```python
from build123d import *

# Parameters (mm, degrees)
PAD_DEPTH         = 27
SKETCH001_R       = 1.6
POCKET_DEPTH      = 14.501
POCKET_DEPTH_BACK = -14.501


with BuildPart() as part:
    # Sketch → Pad (new body, symmetric)
    with BuildSketch(Plane.XZ):
        Polygon((-14.5, 14.1), (-14.5, 0), (14.5, 0), (14.5, 14.1), (12.95, 14.1), (12.95, 1.2), (-12.95, 1.2), (-12.95, 14.1), align=None)
    extrude(amount=PAD_DEPTH, both=True)

    # Sketch001 → Pocket (cut, two sides)
    with BuildSketch(Plane.YZ) as pocket_sk:
        with Locations((-12.5, 9.1)):
            Circle(SKETCH001_R)
        with Locations((12.5, 9.1)):
            Circle(SKETCH001_R)
    extrude(amount=-POCKET_DEPTH, mode=Mode.SUBTRACT)
    extrude(pocket_sk.sketch, amount=-POCKET_DEPTH_BACK, mode=Mode.SUBTRACT)


solid = part.part
```
The listing builds one solid part. Answer for the finished solid, in the listing's coordinates (mm). A direction names the side the tool comes from. Round coordinates to 2 decimals unless told otherwise and drop trailing zeros. Order: outer loops, then holes, each group sorted by start corner. A loop starts at its lowest first (then second) coordinate and runs counter-clockwise, first axis right, second up. Notation, with made-up numbers: (59, -4) -> (74, -4) arc R30 cw to (74, 32) -> close; hole circle Ø5 at (35, 87.5). An arc over 180 degrees is marked (long way). Answer as CSV lines item,"result". Start each with the question number.
(1) A tool of negligible diameter and unlimited length cuts with its end or side. For faces 4 (the face through (0, 0, 1.2)), 5 (the face through (-2, -27, 1)), from which of +Z, -Z, +X, -X, +Y, -Y can it reach the whole face along a straight path? Write none if from no direction.
(2) For a pull along X with two mould halves and no side action, classify faces 1 (the face through (-14, 0, 14.1)), 2 (the face through (12.95, 0, 8)), 3 (the face through (-14.5, 0, 7)) as +X half, -X half, draft (parallel to the pull), parting line (faces both ways), or undercut.
(3) The part is cut by section D-D (x = 11.25). Determine the outline of the cut face in (y, z), then the cut area to 3 significant figures.
(4) The part is cut by section A-A (z = 9.1). Determine the outline of the cut face in (x, y), then the cut area to 3 significant figures.
(5) Find the intervals of material crossed by probe 1 along Y at (x, z) = (13.7, 9.1); probe 2 along X at (y, z) = (19, 5); probe 3 along Z at (x, y) = (13.5, -12.5), in increasing order. Write a range as from..to.
(6) A flat-ended cylindrical pin translates along its axis: pin 1 Ø1.5 at (x, y) = (-5.5, -13) entering from +Z. Find the tip coordinate at first contact, or state that the pin passes through.
(7) The part is cut by section C-C (y = 4). Determine the outline of the cut face in (x, z), then the cut area to 3 significant figures.
(8) The part is cut by section B-B (y = 12.5). Determine the outline of the cut face in (x, z).
Evaluation:
1,face 4,"+Z, +Y, -Y"
1,face 5,"+Z, -Z, +X, -X, -Y"
2,face 1,"draft"
2,face 2,"undercut"
2,face 3,"-X half"
3,outline,"(-27, 0) -> (27, 0) -> (27, 1.2) -> (-27, 1.2) -> close"
3,area,"64.8 mm²"
4,outline,"(-14.5, -27) -> (-12.95, -27) -> (-12.95, -14.1) -> (-14.5, -14.1) -> close; (-14.5, -10.9) -> (-12.95, -10.9) -> (-12.95, 10.9) -> (-14.5, 10.9) -> close; (-14.5, 14.1) -> (-12.95, 14.1) -> (-12.95, 27) -> (-14.5, 27) -> close; (12.95, -27) -> (14.5, -27) -> (14.5, -14.1) -> (12.95, -14.1) -> close; (12.95, -10.9) -> (14.5, -10.9) -> (14.5, 10.9) -> (12.95, 10.9) -> close; (12.95, 14.1) -> (14.5, 14.1) -> (14.5, 27) -> (12.95, 27) -> close"
4,area,"148 mm²"
5,probe 1,"-27..-14.1, -10.9..10.9, 14.1..27"
5,probe 2,"-14.5..-12.95, 12.95..14.5"
5,probe 3,"0..7.5, 10.7..14.1"
6,pin 1,"z = 1.2"
7,outline,"(-14.5, 0) -> (14.5, 0) -> (14.5, 14.1) -> (12.95, 14.1) -> (12.95, 1.2) -> (-12.95, 1.2) -> (-12.95, 14.1) -> (-14.5, 14.1) -> close"
7,area,"74.8 mm²"
8,outline,"(-14.5, 0) -> (14.5, 0) -> (14.5, 7.5) -> (12.95, 7.5) -> (12.95, 1.2) -> (-12.95, 1.2) -> (-12.95, 7.5) -> (-14.5, 7.5) -> close; (-14.5, 10.7) -> (-12.95, 10.7) -> (-12.95, 14.1) -> (-14.5, 14.1) -> close; (12.95, 10.7) -> (14.5, 10.7) -> (14.5, 14.1) -> (12.95, 14.1) -> close"
